For this review, use the dimensioned drawing (mm, ordinates from the lowest corner) and the shaded views. Give positions to 0.01 mm unless a question says otherwise; leave off trailing zeros. Loops run counter-clockwise (first coordinate to the right, second up) from the corner with the lowest first, then second, coordinate; pieces in that order, holes last. Notation, with made-up numbers: (-7.75, 16.5) -> (47.25, 16.5) arc R29 cw to (47.25, 36.5) -> close; hole circle Ø11 at (87.5, 55.5). An arc over 180 degrees is marked (long way). Use a Markdown table: item, result. Add a question column.
1. Add section A-A (z = 3.75). State the section outline as (x, y) points.
2. To check wall thickness, follow line 1 (Y direction, x = 3.1, z = 2.25) (1 decimal); line 2 (Y direction, x = 3.25, z = 3.75) (1 decimal); line 3 (X direction, y = 1.75, z = 6.25) (1 decimal). State the ranges of each line that lie inside material, in increasing order.
3. Draft analysis for pull direction Y (two halves, no side actions). For the marked faces 1, 2 and 3, state which applies: pulls with the +Y half, pulls with the -Y half, needs draft (parallel to the pull), parting line crosses it, or undercut.
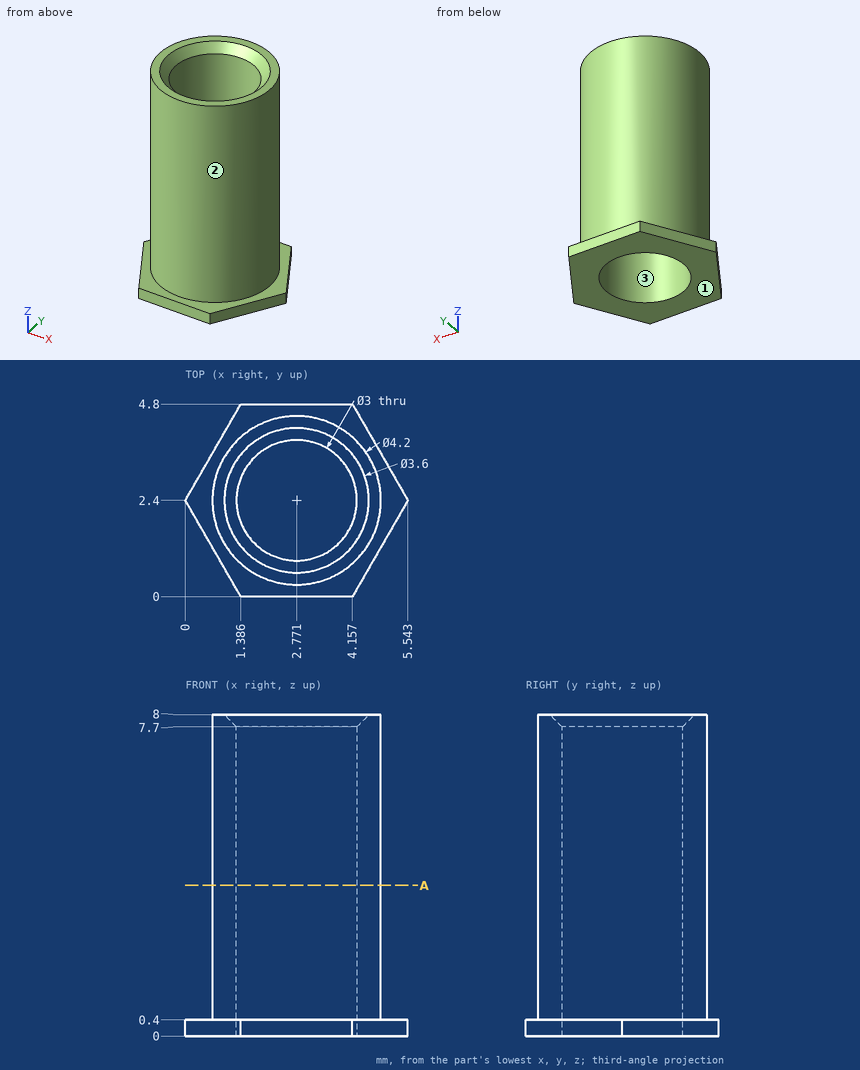
Taken from the geometry:
| question | item | result |
|---|---|---|
| 1 | outline | circle Ø4.2 at (2.77, 2.4); hole circle Ø3 at (2.77, 2.4) |
| 2 | line 1 | y = 0.3 to 0.9, 3.9 to 4.5 |
| 2 | line 2 | y = 0.4 to 1, 3.8 to 4.4 |
| 2 | line 3 | x = 0.8 to 1.4, 4.1 to 4.8 |
| 3 | face 1 | needs draft |
| 3 | face 2 | parting line crosses it |
| 3 | face 3 | undercut |
